Autodesk Inventor part; units mm, degrees
ref_plane "YZ Plane" through (0, 0, 0) normal (1, 0, 0) x (0, 1, 0)
ref_plane "XZ Plane" through (0, 0, 0) normal (0, 1, 0) x (-1, 0, 0)
ref_plane "XY Plane" through (0, 0, 0) normal (0, 0, 1) x (1, 0, 0)
sketch "Sketch1" plane through (0, 0, 0) normal (0, 1, 0) x (-1, 0, 0)
  line L0 (0, 0) -> (76.2, 0)
  line L1 (76.2, 0) -> (76.2, -114.3)
  line L2 (76.2, -114.3) -> (0, -114.3)
  line L3 (0, -114.3) -> (0, 0)
  dimension "d0" = 76.2
  dimension "d1" = 114.3
extrude "Extrusion1" add sketch "Sketch1" along normal blind 3.175
hole "Hole1" at (-9.525, 3.175, -9.525) direction (0, -1, 0) diameter 6.35 depth 25.4 tip angle 118
hole "Hole2" at (-9.525, 3.175, -104.775) direction (0, -1, 0) diameter 6.35 depth 25.4 tip angle 118
hole "Hole3" at (-66.675, 3.175, -104.775) direction (0, -1, 0) diameter 6.35 depth 25.4 tip angle 118
hole "Hole4" at (-66.675, 3.175, -9.525) direction (0, -1, 0) diameter 6.35 depth 25.4 tip angle 118
hole "Hole5" at (-38.1, 3.175, -88.9) direction (0, -1, 0) diameter 28.575 depth 25.4 tip angle 118
hole "Hole6" at (-38.1, 3.175, -38.1) direction (0, -1, 0) diameter 9.525 depth 25.4 tip angle 118
hole "Hole7" at (-38.1, 3.175, -12.4968) direction (0, -1, 0) diameter 4.0386 depth 25.4 tip angle 118
hole "Hole8" at (-38.1, 3.175, -63.7032) direction (0, -1, 0) diameter 4.0386 depth 25.4 tip angle 118
properties part number "Gearbox plate"
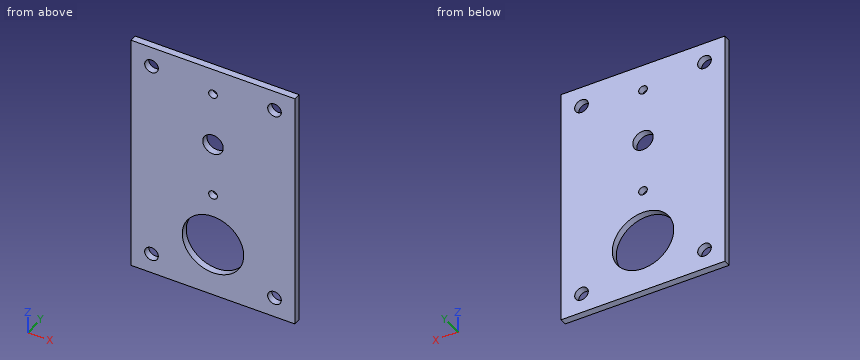
Verification items for the finished model (mm, model axes). Give positions to 0.01 mm unless a question says otherwise; leave off trailing zeros. Loops run counter-clockwise (first coordinate to the right, second up) from the corner with the lowest first, then second, coordinate; pieces in that order, holes last. Notation, with made-up numbers: (44.5, 70.5) - (99.5, 70.5) arc R23 ccw to (99.5, 92.5) - close; hole circle Ø10 at (-31.75, 21.5). An arc over 180 degrees is marked (long way). Write item = value, one per line. Start each with the question number.
Q1. Thickness scan on line 1 (Z direction, x = -38.1, y = 1.3); line 2 (Z direction, x = -36, y = 0.6); line 3 (Z direction, x = -40.5, y = 2.15). Record the ranges inside material, lowest first.
Q2. Cross-section at B-B, the plane x = -34.5. Enter the section's corners in (y, z) (3 decimals).
Q3. Cross-section at C-C, the plane y = 1.8. State how many separate pieces and enclosed holes the cut face has, and give its area (3 significant figures).
Q4. Cross-section at A-A, the plane z = -88.9. Enter the section's corners in (x, y) (1 decimal), and give its area (3 significant figures).
Q5. Cross-section at D-D, the plane z = -38.1. Enter the section's corners in (x, y) (1 decimal).
Answer key:
q1.line_1 = -114.3 to -103.19, -74.61 to -65.72, -61.68 to -42.86, -33.34 to -14.52, -10.48 to 0
q1.line_2 = -114.3 to -103.03, -74.77 to -42.37, -33.83 to 0
q1.line_3 = -114.3 to -102.98, -74.82 to -42.21, -33.99 to 0
q2.outline = (0, -114.3) - (3.175, -114.3) - (3.175, -102.727) - (0, -102.727) - close; (0, -75.073) - (3.175, -75.073) - (3.175, -41.218) - (0, -41.218) - close; (0, -34.982) - (3.175, -34.982) - (3.175, 0) - (0, 0) - close
q3.separate_pieces = 1
q3.enclosed_holes = 8
q3.area = 7,840 mm^2
q4.outline = (-76.2, 0) - (-52.4, 0) - (-52.4, 3.2) - (-76.2, 3.2) - close; (-23.8, 0) - (0, 0) - (0, 3.2) - (-23.8, 3.2) - close
q4.area = 151 mm^2
q5.outline = (-76.2, 0) - (-42.9, 0) - (-42.9, 3.2) - (-76.2, 3.2) - close; (-33.3, 0) - (0, 0) - (0, 3.2) - (-33.3, 3.2) - close
